```python
from build123d import *

# Parameters (mm, degrees)
F0_R     = 9.5
F1_DEPTH = 5
F2_R     = 1.5
F2_R_2   = 1
F3_DEPTH = 5.001
F4_R     = 1
F5_DEPTH = 25


with BuildPart() as f1:
    # F0 (on Front) → F1 (new body)
    with BuildSketch(Plane.XZ):
        Circle(F0_R)
    extrude(amount=-F1_DEPTH)

    # F2 (on face) → F3 (cut, through all)
    with BuildSketch(Plane.XZ):
        Circle(F2_R)
        with Locations((0, -6)):
            Circle(F2_R_2)
    extrude(amount=-F3_DEPTH, mode=Mode.SUBTRACT)

    # F4 (on Top) → F5 (cut)
    with BuildSketch(Plane.XY):
        with Locations((0, 2.5)):
            Circle(F4_R)
    extrude(amount=F5_DEPTH, mode=Mode.SUBTRACT)


solid = f1.part
```
Geometry: final body of the model. Coordinates: model frame, mm. Round coordinates to 2 decimals unless told otherwise and drop trailing zeros. Write each loop counter-clockwise with the first axis right and the second up, starting at its lowest first coordinate (ties: lowest second). Pieces come first, ordered by that corner, then holes.
Item 1: Pin query (flat end, axial travel): P1, Ø5, axis at x = 4.5, z = -1, coming from the -Y side; P2, Ø1, axis at x = 4.5, y = 4, coming from the -Z side. Return the tip coordinate at first contact, or that it passes through.
Item 2: Material intervals for L1, parallel to Z at x = 0, y = 3.55; L2, parallel to Z at x = 0, y = 2.8; L3, parallel to Y at x = 0, z = 4.5, sorted ascending.
Item 3: Section query D-D (z = 8.25). Return loops of the section in (x, y), plus the area to 3 significant figures.
Item 4: Mould query, pull axis Z, two halves, no side actions, for faces 1 (the face through (-0.13, 3.49, 5.25)), 2 (the face through (4.38, 2.46, -8.43)), 3 (the face through (-0.325, 2.465, -1.464)). Classes: +Z half, -Z half, draft (parallel to the pull), parting line (faces both ways), or undercut.
Item 5: Section query C-C (y = 4.3). Return loops of the section in (x, z), plus the area to 3 significant figures.
Item 6: Section query B-B (z = -6.75). Return loops of the section in (x, y).
Item 7: Section query A-A (x = 0). Return loops of the section in (y, z).
Completed:
1. P1: stops at y = 0
1. P2: stops at z = -8.62
2. L1: z = -9.5 to -7, -5 to -1.5, 1.5 to 9.5
2. L2: z = -9.5 to -7, -5 to -1.5
2. L3: y = 0 to 1.5, 3.5 to 5
3. outline: (-4.71, 0) - (4.71, 0) - (4.71, 5) - (-4.71, 5) - close; hole circle Ø2 at (0, 2.5)
3. area: 44.0 mm2
4. face 1: draft
4. face 2: parting line
4. face 3: undercut
5. outline: circle Ø19 at (0, 0); hole circle Ø3 at (0, 0); hole circle Ø2 at (0, -6)
5. area: 273 mm2
6. outline: (-6.68, 0) - (-0.66, 0) - (-0.66, 5) - (-6.68, 5) - close; (0.66, 0) - (6.68, 0) - (6.68, 5) - (0.66, 5) - close
7. outline: (0, -9.5) - (5, -9.5) - (5, -7) - (0, -7) - close; (0, -5) - (5, -5) - (5, -1.5) - (0, -1.5) - close; (0, 1.5) - (1.5, 1.5) - (1.5, 9.5) - (0, 9.5) - close; (3.5, 1.5) - (5, 1.5) - (5, 9.5) - (3.5, 9.5) - close
